Read the model definition and answer for the solid it produces. Units are mm, in the model's axes. A direction names the side the tool comes from. Coordinates: 2 decimals unless noted, no trailing zeros. Write each loop counter-clockwise with the first axis right and the second up, starting at its lowest first coordinate (ties: lowest second). Pieces come first, ordered by that corner, then holes. Notation, with made-up numbers: M 75.25,7 L 108.25,7 A8 cw 108.25,19 Z; hole C 46,75.5 d5. An arc over 180 degrees is marked long. Write item = value, one per line.
from build123d import *

# Parameters (mm, degrees)
F1_R         = 140.9846966486
F2_DEPTH     = 400
F3_DEPTH     = 25
F4_T1_DEPTH  = 2182.8427124746
F4_T6_DEPTH  = 1431.9836481951
F4_S7_R      = 140.9846966486
F4_T8_DEPTH  = 728
F4_T12_DEPTH = 1181.3708498985
F4_S13_R     = 140.9846966486
F4_T14_DEPTH = 602
F4_T19_DEPTH = 1431.9836481951
F4_S20_R     = 140.9846966486
F4_T21_DEPTH = 728
F4_T25_DEPTH = 1700
F4_T31_DEPTH = 1181.3708498985
F4_S32_R     = 140.9846966486
F4_T33_DEPTH = 602
F4_T38_DEPTH = 1181.3708498985
F4_S39_R     = 140.9846966486
F4_T40_DEPTH = 602
F4_T45_DEPTH = 1431.9836481951
F4_S46_R     = 140.9846966486
F4_T47_DEPTH = 728
F4_T52_DEPTH = 1700
F4_T56_DEPTH = 1181.3708498985
F4_T63_DEPTH = 1231.3708498985
F4_S64_R     = 140.9846966486
F4_T65_DEPTH = 627
F4_T69_DEPTH = 1231.3708498985
F4_S70_R     = 140.9846966486
F4_T71_DEPTH = 627
F4_T78_DEPTH = 1700
F4_T82_DEPTH = 1181.3708498985
F5_R         = 5


# Not quite as in the source:
# - a fillet or chamfer that OpenCascade refuses, or shapes differently, is made with other operations: its cross-section is extruded or revolved along the edge and cut away or added


with BuildPart() as f2:
    # F1 (on face) → F2 (new body, symmetric)
    with BuildSketch(Plane.XZ):
        with Locations((0, 941.6702985764)):
            Circle(F1_R)
    extrude(amount=F2_DEPTH, both=True)

    # F0 (on Front) → F3 (join, symmetric)
    with BuildSketch(Plane.XZ):
        Polygon((0, -100), (1041.4213562373, -100), (0, 941.4213562373), (-1041.4213562373, -100), align=None)
        Polygon((800, 0), (0, 0), (-800, 0), (0, 800), align=None, mode=Mode.SUBTRACT)
    extrude(amount=F3_DEPTH, both=True)

    # F4: fillet of radius 20 on 8 edges, made by hand

    # F4_s2 → F4_t1 (cut)
    with BuildSketch(Plane.YZ.offset(-1091.4213562373)):
        with BuildLine():
            ThreePointArc((-25, -80), (-19.1421356237, -94.1421356237), (-5, -100))
            Line((-5, -100), (-25, -100))
            Line((-25, -100), (-25, -80))
        make_face()
    extrude(amount=F4_T1_DEPTH, mode=Mode.SUBTRACT)


with BuildPart() as f4_tool4:
    # F4_s5 → F4_t6 (new body)
    with BuildSketch(Plane(origin=(406.4993310091, 0, 406.4993310091), x_dir=(0, 1, 0), z_dir=(-0.7071067812, 0, -0.7071067812))):
        with BuildLine():
            ThreePointArc((-25, -645.6854249492), (-19.1421356237, -659.827560573), (-5, -665.6854249492))
            Line((-5, -665.6854249492), (-25, -665.6854249492))
            Line((-25, -665.6854249492), (-25, -645.6854249492))
        make_face()
    extrude(amount=F4_T6_DEPTH)

    # F4_s7 → F4_t8 (cut, symmetric)
    with BuildSketch(Plane.XZ.offset(15)):
        with Locations((0, 941.6702985764)):
            Circle(F4_S7_R)
    extrude(amount=F4_T8_DEPTH, both=True, mode=Mode.SUBTRACT)


with BuildPart() as f2_1:
    add(f2.part)

    # F4_t3: cut F4_tool4
    add(f4_tool4.part, mode=Mode.SUBTRACT)


with BuildPart() as f4_tool10:
    # F4_s11 → F4_t12 (new body)
    with BuildSketch(Plane(origin=(-435.3553390593, 0, -435.3553390593), x_dir=(0, 1, 0), z_dir=(0.7071067812, 0, 0.7071067812))):
        with BuildLine():
            ThreePointArc((-25, 585.6854249492), (-19.1421356237, 571.5432893255), (-5, 565.6854249492))
            Line((-5, 565.6854249492), (-25, 565.6854249492))
            Line((-25, 565.6854249492), (-25, 585.6854249492))
        make_face()
    extrude(amount=F4_T12_DEPTH)

    # F4_s13 → F4_t14 (cut, symmetric)
    with BuildSketch(Plane.XZ.offset(15)):
        with Locations((0, 941.6702985764)):
            Circle(F4_S13_R)
    extrude(amount=F4_T14_DEPTH, both=True, mode=Mode.SUBTRACT)

    split(bisect_by=Plane.XY, keep=Keep.TOP)


with BuildPart() as f2_2:
    add(f2_1.part)

    # F4_t9: cut F4_tool10
    add(f4_tool10.part, mode=Mode.SUBTRACT)


with BuildPart() as f4_tool17:
    # F4_s18 → F4_t19 (new body)
    with BuildSketch(Plane(origin=(406.4993310091, 0, 406.4993310091), x_dir=(0, 1, 0), z_dir=(-0.7071067812, 0, -0.7071067812))):
        with BuildLine():
            ThreePointArc((25, -645.6854249492), (19.1421356237, -659.827560573), (5, -665.6854249492))
            Line((5, -665.6854249492), (25, -665.6854249492))
            Line((25, -665.6854249492), (25, -645.6854249492))
        make_face()
    extrude(amount=F4_T19_DEPTH)

    # F4_s20 → F4_t21 (cut, symmetric)
    with BuildSketch(Plane.XZ.offset(-15)):
        with Locations((0, 941.6702985764)):
            Circle(F4_S20_R)
    extrude(amount=F4_T21_DEPTH, both=True, mode=Mode.SUBTRACT)


with BuildPart() as f2_3:
    add(f2_2.part)

    # F4_t16: cut F4_tool17
    add(f4_tool17.part, mode=Mode.SUBTRACT)


with BuildPart() as f4_tool23:
    # F4_s24 → F4_t25 (new body)
    with BuildSketch(Plane.YZ.offset(850)):
        with BuildLine():
            ThreePointArc((-25, -20), (-19.1421356237, -5.8578643763), (-5, 0))
            Line((-5, 0), (-25, 0))
            Line((-25, 0), (-25, -20))
        make_face()
    extrude(amount=-F4_T25_DEPTH)

    split(bisect_by=Plane(origin=(-400, 0, 400), x_dir=(0, 1, 0), z_dir=(0.7071067812, 0, -0.7071067812)), keep=Keep.TOP)

    split(bisect_by=Plane(origin=(400, 0, 400), x_dir=(0, 1, 0), z_dir=(-0.7071067812, 0, -0.7071067812)), keep=Keep.TOP)


with BuildPart() as f2_4:
    add(f2_3.part)

    # F4_t22: cut F4_tool23
    add(f4_tool23.part, mode=Mode.SUBTRACT)


with BuildPart() as f4_tool29:
    # F4_s30 → F4_t31 (new body)
    with BuildSketch(Plane(origin=(-400, 0, 400), x_dir=(0, 1, 0), z_dir=(0.7071067812, 0, -0.7071067812))):
        with BuildLine():
            ThreePointArc((-25, 585.6854249492), (-19.1421356237, 571.5432893255), (-5, 565.6854249492))
            Line((-5, 565.6854249492), (-25, 565.6854249492))
            Line((-25, 565.6854249492), (-25, 585.6854249492))
        make_face()
    extrude(amount=F4_T31_DEPTH)

    # F4_s32 → F4_t33 (cut, symmetric)
    with BuildSketch(Plane.XZ.offset(15)):
        with Locations((0, 941.6702985764)):
            Circle(F4_S32_R)
    extrude(amount=F4_T33_DEPTH, both=True, mode=Mode.SUBTRACT)

    split(bisect_by=Plane.XY, keep=Keep.TOP)


with BuildPart() as f2_5:
    add(f2_4.part)

    # F4_t28: cut F4_tool29
    add(f4_tool29.part, mode=Mode.SUBTRACT)


with BuildPart() as f4_tool36:
    # F4_s37 → F4_t38 (new body)
    with BuildSketch(Plane(origin=(-400, 0, 400), x_dir=(0, 1, 0), z_dir=(0.7071067812, 0, -0.7071067812))):
        with BuildLine():
            ThreePointArc((25, 585.6854249492), (19.1421356237, 571.5432893255), (5, 565.6854249492))
            Line((5, 565.6854249492), (25, 565.6854249492))
            Line((25, 565.6854249492), (25, 585.6854249492))
        make_face()
    extrude(amount=F4_T38_DEPTH)

    # F4_s39 → F4_t40 (cut, symmetric)
    with BuildSketch(Plane.XZ.offset(-15)):
        with Locations((0, 941.6702985764)):
            Circle(F4_S39_R)
    extrude(amount=F4_T40_DEPTH, both=True, mode=Mode.SUBTRACT)

    split(bisect_by=Plane.XY, keep=Keep.TOP)


with BuildPart() as f2_6:
    add(f2_5.part)

    # F4_t35: cut F4_tool36
    add(f4_tool36.part, mode=Mode.SUBTRACT)


with BuildPart() as f4_tool43:
    # F4_s44 → F4_t45 (new body)
    with BuildSketch(Plane(origin=(606.066017178, 0, -606.066017178), x_dir=(0, 1, 0), z_dir=(-0.7071067812, 0, 0.7071067812))):
        with BuildLine():
            ThreePointArc((-5, -665.6854249492), (-19.1421356237, -659.827560573), (-25, -645.6854249492))
            Line((-25, -645.6854249492), (-25, -665.6854249492))
            Line((-25, -665.6854249492), (-5, -665.6854249492))
        make_face()
    extrude(amount=F4_T45_DEPTH)

    # F4_s46 → F4_t47 (cut, symmetric)
    with BuildSketch(Plane.XZ.offset(15)):
        with Locations((0, 941.6702985764)):
            Circle(F4_S46_R)
    extrude(amount=F4_T47_DEPTH, both=True, mode=Mode.SUBTRACT)


with BuildPart() as f2_7:
    add(f2_6.part)

    # F4_t42: cut F4_tool43
    add(f4_tool43.part, mode=Mode.SUBTRACT)


with BuildPart() as f4_tool50:
    # F4_s51 → F4_t52 (new body)
    with BuildSketch(Plane.YZ.offset(850)):
        with BuildLine():
            ThreePointArc((-25, -20), (-19.1421356237, -5.8578643763), (-5, 0))
            Line((-5, 0), (-25, 0))
            Line((-25, 0), (-25, -20))
        make_face()
    extrude(amount=-F4_T52_DEPTH)

    split(bisect_by=Plane(origin=(-400, 0, 400), x_dir=(0, 1, 0), z_dir=(-0.7071067812, 0, 0.7071067812)), keep=Keep.TOP)


with BuildPart() as f4_tool54:
    # F4_s55 → F4_t56 (new body)
    with BuildSketch(Plane(origin=(-435.3553390593, 0, -435.3553390593), x_dir=(0, 1, 0), z_dir=(0.7071067812, 0, 0.7071067812))):
        with BuildLine():
            ThreePointArc((-25, 585.6854249492), (-19.1421356237, 571.5432893255), (-5, 565.6854249492))
            Line((-5, 565.6854249492), (-25, 565.6854249492))
            Line((-25, 565.6854249492), (-25, 585.6854249492))
        make_face()
    extrude(amount=F4_T56_DEPTH)

    split(bisect_by=Plane.XY, keep=Keep.BOTTOM)


with BuildPart() as f4_tool50_1:
    add(f4_tool50.part)

    # F4_t58: intersect F4_tool54
    add(f4_tool54.part, mode=Mode.INTERSECT)


with BuildPart() as f2_8:
    add(f2_7.part)

    # F4_t48: cut F4_tool50
    add(f4_tool50_1.part, mode=Mode.SUBTRACT)


with BuildPart() as f4_tool61:
    # F4_s62 → F4_t63 (new body)
    with BuildSketch(Plane(origin=(-435.3553390593, 0, 435.3553390593), x_dir=(0, 1, 0), z_dir=(0.7071067812, 0, -0.7071067812))):
        with BuildLine():
            ThreePointArc((-25, 585.6854249492), (-19.1421356237, 571.5432893255), (-5, 565.6854249492))
            Line((-5, 565.6854249492), (-25, 565.6854249492))
            Line((-25, 565.6854249492), (-25, 585.6854249492))
        make_face()
    extrude(amount=F4_T63_DEPTH)

    # F4_s64 → F4_t65 (cut, symmetric)
    with BuildSketch(Plane.XZ.offset(15)):
        with Locations((0, 941.6702985764)):
            Circle(F4_S64_R)
    extrude(amount=F4_T65_DEPTH, both=True, mode=Mode.SUBTRACT)

    split(bisect_by=Plane(origin=(-400, 0, 400), x_dir=(0, 1, 0), z_dir=(-0.7071067812, 0, 0.7071067812)), keep=Keep.TOP)


with BuildPart() as f4_tool67:
    # F4_s68 → F4_t69 (new body)
    with BuildSketch(Plane(origin=(-435.3553390593, 0, -435.3553390593), x_dir=(0, 1, 0), z_dir=(0.7071067812, 0, 0.7071067812))):
        with BuildLine():
            ThreePointArc((-25, 585.6854249492), (-19.1421356237, 571.5432893255), (-5, 565.6854249492))
            Line((-5, 565.6854249492), (-25, 565.6854249492))
            Line((-25, 565.6854249492), (-25, 585.6854249492))
        make_face()
    extrude(amount=F4_T69_DEPTH)

    # F4_s70 → F4_t71 (cut, symmetric)
    with BuildSketch(Plane.XZ.offset(15)):
        with Locations((0, 941.6702985764)):
            Circle(F4_S70_R)
    extrude(amount=F4_T71_DEPTH, both=True, mode=Mode.SUBTRACT)

    split(bisect_by=Plane(origin=(400, 0, 400), x_dir=(0, 1, 0), z_dir=(0.7071067812, 0, 0.7071067812)), keep=Keep.TOP)


with BuildPart() as f4_tool61_1:
    add(f4_tool61.part)

    # F4_t73: intersect F4_tool67
    add(f4_tool67.part, mode=Mode.INTERSECT)


with BuildPart() as f2_9:
    add(f2_8.part)

    # F4_t59: cut F4_tool61
    add(f4_tool61_1.part, mode=Mode.SUBTRACT)


with BuildPart() as f4_tool76:
    # F4_s77 → F4_t78 (new body)
    with BuildSketch(Plane.YZ.offset(850)):
        with BuildLine():
            ThreePointArc((-25, -20), (-19.1421356237, -5.8578643763), (-5, 0))
            Line((-5, 0), (-25, 0))
            Line((-25, 0), (-25, -20))
        make_face()
    extrude(amount=-F4_T78_DEPTH)

    split(bisect_by=Plane(origin=(400, 0, 400), x_dir=(0, 1, 0), z_dir=(0.7071067812, 0, 0.7071067812)), keep=Keep.TOP)


with BuildPart() as f4_tool80:
    # F4_s81 → F4_t82 (new body)
    with BuildSketch(Plane(origin=(-400, 0, 400), x_dir=(0, 1, 0), z_dir=(0.7071067812, 0, -0.7071067812))):
        with BuildLine():
            ThreePointArc((-25, 585.6854249492), (-19.1421356237, 571.5432893255), (-5, 565.6854249492))
            Line((-5, 565.6854249492), (-25, 565.6854249492))
            Line((-25, 565.6854249492), (-25, 585.6854249492))
        make_face()
    extrude(amount=F4_T82_DEPTH)

    split(bisect_by=Plane.XY, keep=Keep.BOTTOM)


with BuildPart() as f4_tool76_1:
    add(f4_tool76.part)

    # F4_t84: intersect F4_tool80
    add(f4_tool80.part, mode=Mode.INTERSECT)


with BuildPart() as f2_10:
    add(f2_9.part)

    # F4_t74: cut F4_tool76
    add(f4_tool76_1.part, mode=Mode.SUBTRACT)

    # F5
    f5_edges = [f2_10.edges().sort_by_distance(p)[0] for p in [
        (-140.984697, 400, 941.670299),
        (-140.984697, -400, 941.670299),
    ]]
    fillet(f5_edges, radius=F5_R)


solid = f2_10.part
Item 1: Find section A-A (y = 130.5). Determine the outline of the cut face in (x, z).
Worked answers:
outline = C 0,941.67 d281.97
Item 2: Which of the six approach directions +Z, -Z, +X, -X, +Y, -Y give full straight-line access (tool end or side, diameter ignored) to faces 5 (the face through (-394, 10, 406)), 6 (the face through (405.625, 19.297, 402.881)), 7 (the face through (-2, -400, 944))?
Worked answers:
face_5 = +Y, -Y
face_6 = +Y
face_7 = +Z, -Z, +X, -X, -Y
Item 3: For a pull along X with two mould halves and no side action, classify faces 1 (the face through (9, 25, -11)), 2 (the face through (406, 0, 394)), 3 (the face through (-559.128, 19.297, 373.788)), 4 (the face through (572.548, -18.986, 360.807)) as released by +X, released by -X, zero draft, split by the parting line, or undercut.
Worked answers:
face_1 = zero draft
face_2 = undercut
face_3 = released by -X
face_4 = released by +X
Item 4: Consider line 1 along Y through (x, z) = (-678, -27); line 2 along Y through (x, z) = (-677, 148); line 3 along X through (y, z) = (189.5, 962). Determine where each line is inside the solid, lowest interval first. Write a range as from..to.
Worked answers:
line_1 = -25..25
line_2 = -24.86..25
line_3 = -139.51..139.51
Item 5: Flat-ended cylindrical pins translate along their axes: pin 1 (24 mm diameter, centred on x = -298, y = 16.5, fed in from +Z); pin 2 (1.5 mm diameter, centred on x = -112.5, y = -289.5, fed in from -Z). Find the tip coordinate at first contact, or state that the pin passes through.
Worked answers:
pin_1 = 652.8
pin_2 = 855.71
